from build123d import *

# Parameters (mm, degrees)
ESQUISSE1_W                            = 53.7
ESQUISSE1_H                            = 42
ESQUISSE1_R                            = 1.75
EXTRUSION1_DEPTH                       = 1.5
FRAISAGE_POUR_VIS_T_TE_FRAIS_E_M2_51_D = 2.59999988
ESQUISSE5_W                            = 2
ESQUISSE5_H                            = 15.5
ENL_V_MAT_EXTRU_1_DEPTH                = 56.35964234
ENL_V_MAT_EXTRU_2_REACH                = 57.36


with BuildPart() as part:
    # Esquisse1 → Extrusion1 (new body)
    with BuildSketch(Plane(origin=(0, 0, 0), x_dir=(0, 0, -1), z_dir=(1, 0, 0))):
        with Locations((-24.35, 0)):
            Rectangle(ESQUISSE1_W, ESQUISSE1_H)
        with Locations((0, -17.5)):
            Circle(ESQUISSE1_R, mode=Mode.SUBTRACT)
        with Locations((0, 12.5)):
            Circle(ESQUISSE1_R, mode=Mode.SUBTRACT)
    extrude(amount=EXTRUSION1_DEPTH)

    # Fraisage pour vis à tête fraisée M2.51 (through all)
    with Locations(Plane(origin=(1.5, 0, 0), x_dir=(0, 0, -1), z_dir=(1, 0, 0))):
        with Locations((0, 17.5), (0, -12.5), (0, 0)):
            Hole(FRAISAGE_POUR_VIS_T_TE_FRAIS_E_M2_51_D / 2)

    # Esquisse5 → Enlèv. mat.-Extru.1 (cut, through all)
    with BuildSketch(Plane.ZY):
        with Locations((3.5, 9.25)):
            Rectangle(ESQUISSE5_W, ESQUISSE5_H)
    extrude(amount=-ENL_V_MAT_EXTRU_1_DEPTH, mode=Mode.SUBTRACT)

    # Esquisse6 → Enlèv. mat.-Extru.2 (cut, up to next)
    with BuildSketch(Plane(origin=(1.5, 0, 0), x_dir=(0, 0, -1), z_dir=(1, 0, 0)), mode=Mode.PRIVATE) as enl_v_mat_extru_2_sk1:
        Polygon((-51.2, 21), (-51.2, -1), (-46.2, 4), (-10, 4), (-10, 18), (-7, 21), align=None)
    enl_v_mat_extru_2_tool1 = extrude(enl_v_mat_extru_2_sk1.sketch, amount=-ENL_V_MAT_EXTRU_2_REACH, mode=Mode.PRIVATE) & part.part
    # Esquisse6 → Enlèv. mat.-Extru.2 (cut, up to next)
    with BuildSketch(Plane(origin=(1.5, 0, 0), x_dir=(0, 0, -1), z_dir=(1, 0, 0)), mode=Mode.PRIVATE) as enl_v_mat_extru_2_sk2:
        Polygon((-51.2, -21), (-46.2, -21), (-51.2, -16), align=None)
    enl_v_mat_extru_2_tool2 = extrude(enl_v_mat_extru_2_sk2.sketch, amount=-ENL_V_MAT_EXTRU_2_REACH, mode=Mode.PRIVATE) & part.part
    add(enl_v_mat_extru_2_tool1.solids().sort_by_distance((1.5, 12.369901, 30.794406))[0], mode=Mode.SUBTRACT)
    add(enl_v_mat_extru_2_tool2.solids().sort_by_distance((1.5, -19.333333, 49.533333))[0], mode=Mode.SUBTRACT)


solid = part.part
Geometry: final body of the model. Coordinates: model frame, mm. A direction names the side the tool comes from. Coordinates: 2 decimals unless noted, no trailing zeros. Loops run counter-clockwise (first coordinate to the right, second up) from the corner with the lowest first, then second, coordinate; pieces in that order, holes last. Notation, with made-up numbers: (82, -5) - (104, -5) arc R22 ccw to (104, 34) - close; hole circle Ø2 at (-18.5, -33.75). An arc over 180 degrees is marked (long way). One line per question, with ' | ' between items. Start each with the question number.
(1) First-contact query: pin 1 (3 mm diameter, centred on y = -6, z = 12.5, fed in from -X); pin 2 (2.5 mm diameter, centred on y = 17.5, z = 0, fed in from -X). Flat tips, straight axial feed; report the tip coordinate or a pass-through.
(2) Cut plane A-A on y = 12.5. Output: boundary loops of the cut face in (x, z).
(3) Reachability of faces 1 (the flat face through (1, 4, 28)), 2 (the flat face through (1, 9, 4.5)), 3 (the flat face through (1, 0, -2.5)) from +Z, -Z, +X, -X, +Y, -Y: full face, straight path, thin tool, end or side. Return the list, or none.
(4) Ray query, L1, parallel to Y at x = 0.75, z = 0; L2, parallel to Z at x = 0.95, y = -18; L3, parallel to Y at x = 0.75, z = 24. Return the intervals inside material, ascending. Write a range as from..to.
(5) Draft query along Y for faces 4 (the cylindrical face through (0.74, -0.79, -1.03)), 5 (the flat face through (1, 11, 10)), 6 (the flat face through (1, 21, 2)). Return one class per face: +Y half, -Y half, draft (parallel to the pull), parting line (faces both ways), or undercut.
(6) Cut plane B-B on y = 0. Output: boundary loops of the cut face in (x, z), and give its area (4 significant figures).
(7) Cut plane D-D on z = 0. Output: boundary loops of the cut face in (x, y).
(8) Cut plane C-C on x = 0.4. Output: boundary loops of the cut face in (y, z), and give its area (3 significant figures).
Here are the results:
1) pin 1: x = 0 | pin 2: through
2) outline: (0, -2.5) - (1.5, -2.5) - (1.5, -1.75) - (0, -1.75) - close; (0, 1.75) - (1.5, 1.75) - (1.5, 2.5) - (0, 2.5) - close; (0, 4.5) - (1.5, 4.5) - (1.5, 10) - (0, 10) - close
3) face 1: +Z, +X, -X, +Y | face 2: +X, -X | face 3: -Z, +X, -X, +Y, -Y
4) L1: -21..-19.25, -15.75..-13.8, -11.2..-1.3, 1.3..10.75, 14.25..16.2, 18.8..21 | L2: -2.5..-1.68, 1.68..49.2 | L3: -21..4
5) face 4: undercut | face 5: draft | face 6: +Y half
6) outline: (0, -2.5) - (1.5, -2.5) - (1.5, -1.3) - (0, -1.3) - close; (0, 1.3) - (1.5, 1.3) - (1.5, 50.2) - (0, 50.2) - close | area: 75.15 mm²
7) outline: (0, -21) - (1.5, -21) - (1.5, -19.25) - (0, -19.25) - close; (0, -15.75) - (1.5, -15.75) - (1.5, -13.8) - (0, -13.8) - close; (0, -11.2) - (1.5, -11.2) - (1.5, -1.3) - (0, -1.3) - close; (0, 1.3) - (1.5, 1.3) - (1.5, 10.75) - (0, 10.75) - close; (0, 14.25) - (1.5, 14.25) - (1.5, 16.2) - (0, 16.2) - close; (0, 18.8) - (1.5, 18.8) - (1.5, 21) - (0, 21) - close
8) outline: (-21, -2.5) - (21, -2.5) - (21, 7) - (18, 10) - (4, 10) - (4, 46.2) - (-1, 51.2) - (-16, 51.2) - (-21, 46.2) - close; hole circle Ø3.5 at (-17.5, 0); hole circle Ø2.6 at (-12.5, 0); hole circle Ø2.6 at (0, 0); hole (1.5, 2.5) - (17, 2.5) - (17, 4.5) - (1.5, 4.5) - close; hole circle Ø3.5 at (12.5, 0); hole circle Ø2.6 at (17.5, 0) | area: 1,460 mm²
